Source: CAD feature listing. Evaluate the final solid. Frame: model axes, mm. A direction names the side the tool comes from. Coordinates: 2 decimals unless noted, no trailing zeros. Loops run counter-clockwise (first coordinate to the right, second up) from the corner with the lowest first, then second, coordinate; pieces in that order, holes last. Notation, with made-up numbers: (4.25, 12.5) -> (48.25, 12.5) arc R16 ccw to (48.25, 27.5) -> close; hole circle Ø6 at (59.25, 62.25). An arc over 180 degrees is marked (long way). Answer as a JSON object with one key per item and string values. Group by question number.
from build123d import *

# Parameters (mm, degrees)
SKETCH_1_W          = 78
SKETCH_1_H          = 58
EXTRUDE_1_DEPTH     = 28
SKETCH_2_W          = 28
SKETCH_2_H          = 15.2
CUT_EXTRUDE_1_DEPTH = 3
SKETCH_5_R          = 14.972823893
SKETCH_5_W          = 36.008932868
SKETCH_5_H          = 40.760932053
EXTRUDE_4_DEPTH     = 0.5
SKETCH_6_R          = 0.5
CUT_EXTRUDE_2_DEPTH = 5
SKETCH_7_R          = 1
SKETCH_7_W          = 15.2
SKETCH_7_H          = 17
CUT_EXTRUDE_3_DEPTH = 3.5


with BuildPart() as part:
    # 草图1 → 凸台-拉伸1 (new body)
    with BuildSketch(Plane.XY):
        with Locations((39, -29)):
            Rectangle(SKETCH_1_W, SKETCH_1_H)
    extrude(amount=EXTRUDE_1_DEPTH)

    # 草图2 → 切除-拉伸1 (cut)
    with BuildSketch(Plane(origin=(0, 0, 0), x_dir=(1, 0, 0), z_dir=(0, 1, 0))):
        with Locations((56, -15.4)):
            Rectangle(SKETCH_2_W, SKETCH_2_H)
    extrude(amount=-CUT_EXTRUDE_1_DEPTH, mode=Mode.SUBTRACT)

    # 草图5 → 凸台-拉伸4 (add)
    with BuildSketch(Plane.XY.offset(28)):
        with Locations((18.486091334, -31.18136891)):
            Circle(SKETCH_5_R)
        with Locations((55.726307101, -31.18136891)):
            Rectangle(SKETCH_5_W, SKETCH_5_H)
    extrude(amount=EXTRUDE_4_DEPTH)

    # 草图6 → 切除-拉伸2 (cut)
    with BuildSketch(Plane(origin=(0, -3, 0), x_dir=(1, 0, 0), z_dir=(0, 1, 0))):
        with Locations(Location((53.5, -18.5, 0), (0, 0, 270))):
            Circle(SKETCH_6_R)
    extrude(amount=-CUT_EXTRUDE_2_DEPTH, mode=Mode.SUBTRACT)

    # 草图7 → 切除-拉伸3 (cut)
    with BuildSketch(Plane(origin=(78, 0, 0), x_dir=(0, 0, -1), z_dir=(1, 0, 0))):
        with Locations(Location((-17, -36, 0), (0, 0, 90))):
            Circle(SKETCH_7_R)
        with Locations((-15.4, -24.5)):
            Rectangle(SKETCH_7_W, SKETCH_7_H)
    extrude(amount=-CUT_EXTRUDE_3_DEPTH, mode=Mode.SUBTRACT)


solid = part.part
1. Section query B-B on z = 17. Return loops of the section in (x, y), then the cut area to 3 significant figures.
2. Pin query (flat end, axial travel): pin 1 Ø4.5 at (x, z) = (58, 17) entering from +Y; pin 2 Ø4 at (x, y) = (12, -9.5) entering from +Z; pin 3 Ø4.5 at (y, z) = (-27.5, 19) entering from +X. Return the tip coordinate at first contact, or that it passes through.
3. Mould query, pull axis Z, two halves, no side actions, for faces 6 (the face through (56, -1, 7.8)), 7 (the face through (0, -29, 14)), 8 (the face through (76, -25, 23)), 9 (the face through (55, -31, 28.5)). Classes: pulls with the +Z half, pulls with the -Z half, needs draft (parallel to the pull), parting line crosses it, or undercut.
4. Section query C-C on y = -20. Return loops of the section in (x, z).
5. Reachability of faces 1 (the face through (76, -25, 7.8)), 2 (the face through (38, -29, 0)), 3 (the face through (18, -31, 28.5)), 4 (the face through (25.395, -44.465, 28.246)), 5 (the face through (70, -1, 16)) from +Z, -Z, +X, -X, +Y, -Y: full face, straight path, thin tool, end or side. Return the list, or none.
6. Section query A-A on x = 66.5. Return loops of the section in (y, z), then the cut area to 3 significant figures.
7. Ray query, L1, parallel to X at y = -5.3, z = 18.5; L2, parallel to Z at x = 53.5, y = -6.4; L3, parallel to Z at x = 77, y = -36. Return the intervals inside material, ascending.
8. Section query D-D on z = 21.25. Return loops of the section in (x, y).
Solved:
{
 "1": {"outline": "(0, -58) -> (78, -58) -> (78, -37) -> (74.5, -37) -> (74.5, -35) -> (78, -35) -> (78, -33) -> (74.5, -33) -> (74.5, -16) -> (78, -16) -> (78, 0) -> (70, 0) -> (70, -3) -> (42, -3) -> (42, 0) -> (0, 0) -> close", "area": "4,370 mm^2"},
 "2": {"pin 1": "y = -3", "pin 2": "z = 28", "pin 3": "x = 74.5"},
 "3": {"face 6": "undercut", "face 7": "needs draft", "face 8": "undercut", "face 9": "pulls with the +Z half"},
 "4": {"outline": "(0, 0) -> (78, 0) -> (78, 7.8) -> (74.5, 7.8) -> (74.5, 23) -> (78, 23) -> (78, 28) -> (73.73, 28) -> (73.73, 28.5) -> (37.72, 28.5) -> (37.72, 28) -> (28.44, 28) -> (28.44, 28.5) -> (8.53, 28.5) -> (8.53, 28) -> (0, 28) -> close"},
 "5": {"face 1": "+X", "face 2": "-Z, +X, -X, +Y, -Y", "face 3": "+Z, +X, -X, +Y, -Y", "face 4": "+Z", "face 5": "+Y"},
 "6": {"outline": "(-58, 0) -> (0, 0) -> (0, 7.8) -> (-3, 7.8) -> (-3, 23) -> (0, 23) -> (0, 28) -> (-10.8, 28) -> (-10.8, 28.5) -> (-51.56, 28.5) -> (-51.56, 28) -> (-58, 28) -> close", "area": "1,600 mm^2"},
 "7": {"L1": "0 to 53, 54 to 78", "L2": "0 to 18, 19 to 28", "L3": "0 to 16, 18 to 28"},
 "8": {"outline": "(0, -58) -> (78, -58) -> (78, -33) -> (74.5, -33) -> (74.5, -16) -> (78, -16) -> (78, 0) -> (70, 0) -> (70, -3) -> (42, -3) -> (42, 0) -> (0, 0) -> close"}
}
